```python
from build123d import *

# Parameters (mm, degrees)
SKETCH3_W                                         = 20
SKETCH3_H                                         = 60
SKETCH3_H_2                                       = 16.009607205
BOSS_EXTRUDE1_DEPTH                               = 50
SKETCH4_W                                         = 16.009607205
SKETCH4_H                                         = 30
CUT_EXTRUDE1_DEPTH                                = 10
FILLET4_R                                         = 15
CSK_FOR_8_FLAT_HEAD_MACHINE_SCREW_100_D           = 4.4958
CSK_FOR_8_FLAT_HEAD_MACHINE_SCREW_100_CSINK_D     = 8.4328
CSK_FOR_8_FLAT_HEAD_MACHINE_SCREW_100_CSINK_ANGLE = 100
SKETCH7_R                                         = 2.5
CUT_EXTRUDE2_DEPTH                                = 30


with BuildPart() as part:
    # Sketch3 → Boss-Extrude1 (new body)
    with BuildSketch(Plane(origin=(0, 0, 0), x_dir=(1, 0, 0), z_dir=(0, 1, 0))):
        Rectangle(SKETCH3_W, SKETCH3_H)
        with Locations((20, 21.995196398)):
            Rectangle(SKETCH3_W, SKETCH3_H_2)
    extrude(amount=BOSS_EXTRUDE1_DEPTH)

    # Sketch4 → Cut-Extrude1 (cut)
    with BuildSketch(Plane(origin=(30, 0, 0), x_dir=(0, 0, -1), z_dir=(1, 0, 0))):
        with Locations((21.995196398, 25)):
            Rectangle(SKETCH4_W, SKETCH4_H)
    extrude(amount=-CUT_EXTRUDE1_DEPTH, mode=Mode.SUBTRACT)

    # Fillet4
    # the kernel refuses this fillet: 15 mm, written as the material it adds along each edge
    with BuildSketch(Plane(origin=(20, 10, -30), x_dir=(1, 0, 0), z_dir=(0, 0, 1))) as fillet4_piece_1:
        with BuildLine():
            CenterArc((15, 14.142135624), FILLET4_R, 180, 70.528779366)
            Line((0, 14.142135624), (-0.3, 14.142135624))
            Line((-0.3, 14.142135624), (-0.3, 0))
            Line((-0.3, 0), (0, -0.3))
            ThreePointArc((0, -0.3), (5, -0.3), (9.9, -0.282842712))
            Line((9.9, -0.282842712), (10, 0))
        make_face()
    extrude(amount=16.009607205)
    with BuildSketch(Plane(origin=(20, 40, -13.990392795), x_dir=(0, -1, 0), z_dir=(0, 0, -1))) as fillet4_piece_2:
        with BuildLine():
            CenterArc((14.142135624, -15), FILLET4_R, 90, 70.528779366)
            Line((0, -10), (-0.282842712, -9.9))
            ThreePointArc((-0.282842712, -9.9), (-0.3, -5), (-0.3, 0))
            Line((-0.3, 0), (0, 0.3))
            Line((0, 0.3), (14.142135624, 0.3))
            Line((14.142135624, 0.3), (14.142135624, 0))
        make_face()
    extrude(amount=16.009607205)

    # CSK for #8 Flat Head Machine Screw (100)1 (through all)
    with Locations(Plane.ZY.offset(10)):
        with Locations((23.5, 8), (23.5, 42)):
            CounterSinkHole(CSK_FOR_8_FLAT_HEAD_MACHINE_SCREW_100_D / 2, CSK_FOR_8_FLAT_HEAD_MACHINE_SCREW_100_CSINK_D / 2, counter_sink_angle=CSK_FOR_8_FLAT_HEAD_MACHINE_SCREW_100_CSINK_ANGLE)

    # Sketch7 → Cut-Extrude2 (cut)
    with BuildSketch(Plane(origin=(0, 0, -30), x_dir=(-1, 0, 0), z_dir=(0, 0, -1))):
        with Locations((0, 10)):
            Circle(SKETCH7_R)
        with Locations((0, 40)):
            Circle(SKETCH7_R)
    extrude(amount=-CUT_EXTRUDE2_DEPTH, mode=Mode.SUBTRACT)


solid = part.part
```
Geometry: final body of the model. Coordinates: model frame, mm. A direction names the side the tool comes from. Give positions to 0.01 mm unless a question says otherwise; leave off trailing zeros. Loops run counter-clockwise (first coordinate to the right, second up) from the corner with the lowest first, then second, coordinate; pieces in that order, holes last. Notation, with made-up numbers: (88, 66.25) -> (108, 66.25) arc R14 cw to (108, 91.25) -> close; hole circle Ø5 at (14, -28.5). An arc over 180 degrees is marked (long way). Use one line per item in the form item = value.
Item 1: Section query D-D on y = 15. Output: boundary loops of the cut face in (x, z), and give its area (3 significant figures).
A:
outline = (-10, -30) -> (23.11, -30) -> (23.11, -13.99) -> (10, -13.99) -> (10, 30) -> (-10, 30) -> close
area = 1,410 mm^2
Item 2: Section query B-B on z = -21. Output: boundary loops of the cut face in (x, y), and give its area (3 significant figures).
A:
outline = (-10, 0) -> (30, 0) -> (30, 10) arc R15 cw to (20, 24.14) -> (20, 25.86) arc R15 cw to (30, 40) -> (30, 50) -> (-10, 50) -> close; hole circle Ø5 at (0, 10); hole circle Ø5 at (0, 40)
area = 1,740 mm^2
Item 3: Draft query along Z for faces 5 (the face through (0.954, 9.519, 25.157)), 6 (the face through (0.954, 43.519, 25.157)), 7 (the face through (18, 25, -13.99)), 8 (the face through (20, 25, -22)). Return one class per face: pulls with the +Z half, pulls with the -Z half, needs draft (parallel to the pull), parting line crosses it, or undercut.
A:
face_5 = undercut
face_6 = undercut
face_7 = pulls with the +Z half
face_8 = needs draft
Item 4: Section query C-C on x = 25.5. Output: boundary loops of the cut face in (y, z), and give its area (3 significant figures).
A:
outline = (0, -30) -> (12.53, -30) -> (12.53, -13.99) -> (0, -13.99) -> close; (37.47, -30) -> (50, -30) -> (50, -13.99) -> (37.47, -13.99) -> close
area = 401 mm^2
Item 5: Pin query (flat end, axial travel): P1, Ø1, axis at y = 12.5, z = -12.5, coming from the +X side; P2, Ø4.5, axis at x = 0, y = 10, coming from the -Z side; P3, Ø3, axis at y = 34.5, z = -16, coming from the +X side; P4, Ø10, axis at x = 15.5, z = 7, coming from the -Y side. Return the tip coordinate at first contact, or that it passes through.
A:
P1 = 10
P2 = 0
P3 = 23.95
P4 = through
Item 6: Line query: probe 1 along Y at (x, z) = (0, -12); probe 2 along Y at (x, z) = (4, 23.5); probe 3 along Z at (x, y) = (12.5, 41). Output: solid intervals per line, ascending.
A:
probe_1 = 0 to 7.5, 12.5 to 37.5, 42.5 to 50
probe_2 = 0 to 5.75, 10.25 to 39.75, 44.25 to 50
probe_3 = -30 to -13.99
Item 7: Section query A-A on x = 21. Output: boundary loops of the cut face in (y, z), and give its area (3 significant figures).
A:
outline = (0, -30) -> (18.76, -30) -> (18.76, -13.99) -> (0, -13.99) -> close; (31.24, -30) -> (50, -30) -> (50, -13.99) -> (31.24, -13.99) -> close
area = 601 mm^2
Item 8: Access query for faces 1 (the face through (5, 50, -7)), 2 (the face through (10, 25, 8)), 3 (the face through (0, 40, 0)), 4 (the face through (22.678, 34.412, -21.883)). Directions: +Z, -Z, +X, -X, +Y, -Y. A direction counts if a zero-diameter tool reaches every point of the face in a straight line with its end or side. Return the directions, or none.
A:
face_1 = +Z, -Z, +X, -X, +Y
face_2 = +Z, +X, +Y, -Y
face_3 = -Z
face_4 = +Z, -Z, +X
